Autodesk Inventor part; units mm, degrees
ref_plane "YZ Plane" through (0, 0, 0) normal (1, 0, 0) x (0, 1, 0)
ref_plane "XZ Plane" through (0, 0, 0) normal (0, 1, 0) x (-1, 0, 0)
ref_plane "XY Plane" through (0, 0, 0) normal (0, 0, 1) x (1, 0, 0)
sketch "Sketch1" plane through (0, 0, 0) normal (0, 0, 1) x (1, 0, 0)
  circle A0 centre (0, 0) radius 25
  dimension "d0" = 50
extrude "Extrusion1" add sketch "Sketch1" along normal blind 2
sketch "Sketch2" plane through (0, 0, 2) normal (0, 0, 1) x (1, 0, 0)
  circle A0 centre (0, 0) radius 23.75
  circle A1 centre (0, 0) radius 22.5
  dimension "d3" = 47.5
  dimension "d4" = 45
extrude "Extrusion2" add sketch "Sketch2" along normal blind 2
properties part number "tapaCargador"
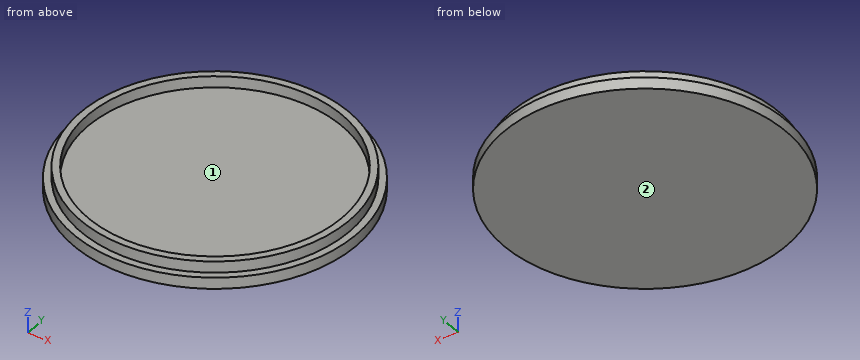
Geometry check sheet. Reference: the model listing, model coordinates, mm. Face numbers are marked on the shaded views. Round coordinates to 2 decimals unless told otherwise and drop trailing zeros. Order: outer loops, then holes, each group sorted by start corner. A loop starts at its lowest first (then second) coordinate and runs counter-clockwise, first axis right, second up. Notation, with made-up numbers: (-24, 70.5) -> (-3, 70.5) arc R33 cw to (-3, 99.5) -> close; hole circle Ø5 at (30.25, -25.75). An arc over 180 degrees is marked (long way). Use one line per item in the form item = value.
1. Mould release check, pull along X, two halves, no side actions. Record for the marked faces 1 and 2: pulls with the +X half, pulls with the -X half, needs draft (parallel to the pull), parting line crosses it, or undercut.
Working result:
face_1 = undercut
face_2 = needs draft
2. Scan lines: line 1 along Y through (x, z) = (0, 3.1); line 2 along Z through (x, y) = (-8, 6); line 3 along X through (y, z) = (-1, 3.5). Record each from-to range of solid material in increasing order. Write a range as from..to.
Working result:
line_1 = -23.75..-22.5, 22.5..23.75
line_2 = 0..2
line_3 = -23.73..-22.48, 22.48..23.73
3. Go/stop test with flat-tipped pins: pin 1 (1 mm diameter, centred on y = -0.5, z = 3, fed in from -X); pin 2 (6 mm diameter, centred on x = 15, y = 4.5, fed in from +Z); pin 3 (1 mm diameter, centred on x = 14.5, z = 1.5, fed in from +Y). Record where each tip stops, or that it passes through.
Working result:
pin_1 = -23.75
pin_2 = 2
pin_3 = 20.71
4. Cross-section at A-A, the plane x = 0. Enter the section's corners in (y, z).
Working result:
outline = (-25, 0) -> (25, 0) -> (25, 2) -> (23.75, 2) -> (23.75, 4) -> (22.5, 4) -> (22.5, 2) -> (-22.5, 2) -> (-22.5, 4) -> (-23.75, 4) -> (-23.75, 2) -> (-25, 2) -> close
5. Cross-section at C-C, the plane z = 0.75. Enter the section's corners in (x, y), plus the area to 3 significant figures.
Working result:
outline = circle Ø50 at (0, 0)
area = 1,960 mm^2
